For this review, take the finished solid that the model builds, in its own axes (mm). Face numbers are marked on the shaded views. Coordinates: 2 decimals unless noted, no trailing zeros. Order: outer loops, then holes, each group sorted by start corner. A loop starts at its lowest first (then second) coordinate and runs counter-clockwise, first axis right, second up. Notation, with made-up numbers: (-17.5, 77) -> (15.5, 77) arc R25 cw to (15.5, 113) -> close; hole circle Ø6 at (64, 10.5). An arc over 180 degrees is marked (long way). Write item = value, one per line. Start each with the question number.
1) Consider section B-B on y = 3.05. Give the boundary of the cut face in (x, z), and give its area (3 significant figures).
2) Consider section C-C on z = -44. Give the boundary of the cut face in (x, y).
3) Draft analysis for pull direction X (two halves, no side actions). For the marked faces 1 and 2, state which applies: +X half, -X half, draft (parallel to the pull), parting line (faces both ways), or undercut.
4) Consider section A-A on x = -34. Give the boundary of the cut face in (y, z), and give its area (3 significant figures).
5) Insertion check: pin 1 Ø4 at (x, z) = (-67, -20.5) entering from +Y. The pin has a flat end and moves straight along its axis. Give the tip position at first contact, or say it passes through.
6) Wall thickness on probe 1 along X at (y, z) = (0.2, -42.5); probe 2 along Z at (x, y) = (-17.5, 1.05); probe 3 along X at (y, z) = (2.9, -38.5): over which ranges is each line inside the solid? List them lowest first. Write a range as [from, to].
7) Consider section D-D on x = -65. Give the boundary of the cut face in (y, z).
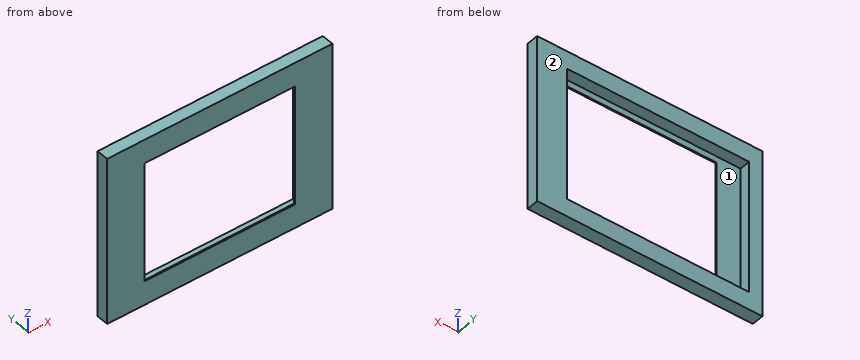
from build123d import *

# Parameters (mm, degrees)
ESBO_O4_W                = 75
ESBO_O4_H                = 56
RESSALTO_EXTRUS_O1_DEPTH = 4
ESBO_O5_W                = 50
ESBO_O5_H                = 40
CORTE_EXTRUS_O1_DEPTH    = 94.685644578
ESBO_O6_W                = 60.7
ESBO_O6_H                = 44.2
CORTE_EXTRUS_O2_DEPTH    = 3.58


with BuildPart() as part:
    # Esboço4 → Ressalto-extrusão1 (new body)
    with BuildSketch(Plane(origin=(0, 0, 0), x_dir=(1, 0, 0), z_dir=(0, 1, 0))):
        with Locations((-37.5, 28)):
            Rectangle(ESBO_O4_W, ESBO_O4_H)
    extrude(amount=RESSALTO_EXTRUS_O1_DEPTH)

    # Esboço5 → Corte-extrusão1 (cut, through all)
    with BuildSketch(Plane(origin=(0, 4, 0), x_dir=(1, 0, 0), z_dir=(0, 1, 0))):
        with Locations((-37.5, 28)):
            Rectangle(ESBO_O5_W, ESBO_O5_H)
    extrude(amount=-CORTE_EXTRUS_O1_DEPTH, mode=Mode.SUBTRACT)

    # Esboço6 → Corte-extrusão2 (cut)
    with BuildSketch(Plane(origin=(0, 4, 0), x_dir=(1, 0, 0), z_dir=(0, 1, 0))):
        with Locations((-40.25, 28)):
            Rectangle(ESBO_O6_W, ESBO_O6_H)
    extrude(amount=-CORTE_EXTRUS_O2_DEPTH, mode=Mode.SUBTRACT)


solid = part.part
Answer sheet:
q1.outline = (-75, -56) -> (0, -56) -> (0, 0) -> (-75, 0) -> close; hole (-70.6, -50.1) -> (-9.9, -50.1) -> (-9.9, -5.9) -> (-70.6, -5.9) -> close
q1.area = 1,520 mm2
q2.outline = (-75, 0) -> (-62.5, 0) -> (-62.5, 0.42) -> (-70.6, 0.42) -> (-70.6, 4) -> (-75, 4) -> close; (-12.5, 0) -> (0, 0) -> (0, 4) -> (-9.9, 4) -> (-9.9, 0.42) -> (-12.5, 0.42) -> close
q3.face_1 = undercut
q3.face_2 = draft
q4.outline = (0, -56) -> (4, -56) -> (4, -50.1) -> (0.42, -50.1) -> (0.42, -48) -> (0, -48) -> close; (0, -8) -> (0.42, -8) -> (0.42, -5.9) -> (4, -5.9) -> (4, 0) -> (0, 0) -> close
q4.area = 49.0 mm2
q5.pin_1 = 0.42
q6.probe_1 = [-75, -62.5], [-12.5, 0]
q6.probe_2 = [-56, -50.1], [-5.9, 0]
q6.probe_3 = [-75, -70.6], [-9.9, 0]
q7.outline = (0, -56) -> (4, -56) -> (4, -50.1) -> (0.42, -50.1) -> (0.42, -5.9) -> (4, -5.9) -> (4, 0) -> (0, 0) -> close
